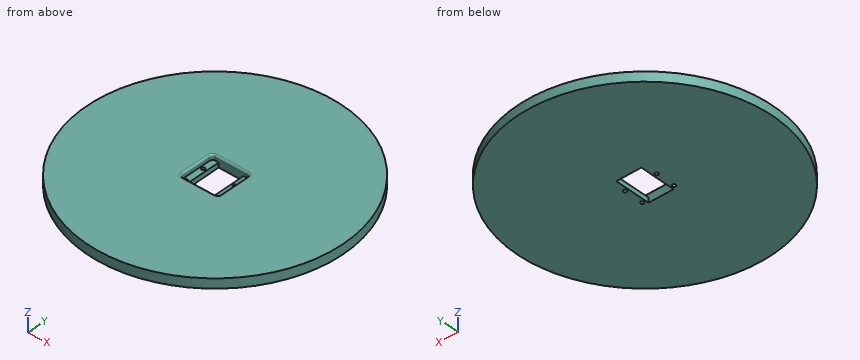
from build123d import *

# Parameters (mm, degrees)
SKETCH1_R           = 84.93125
BOSS_EXTRUDE1_DEPTH = 6.35
CUT_EXTRUDE2_DEPTH  = 3.175
SKETCH4_R           = 1.143
SKETCH4_W           = 16.6116
SKETCH4_H           = 23.7998
CUT_EXTRUDE3_DEPTH  = 3.175
FILLET1_R           = 1.27


with BuildPart() as part:
    # Sketch1 → Boss-Extrude1 (new body)
    with BuildSketch(Plane.XY):
        Circle(SKETCH1_R)
    extrude(amount=BOSS_EXTRUDE1_DEPTH)

    # Sketch2 → Cut-Extrude2 (cut)
    with BuildSketch(Plane.XY.offset(6.35)):
        with BuildLine():
            Line((10.541, 11.8999), (-10.541, 11.8999))
            ThreePointArc((-10.541, 11.8999), (-11.995801492, 11.297301492), (-12.5984, 9.8425))
            Line((-12.5984, 9.8425), (-12.5984, -9.8425))
            ThreePointArc((-12.5984, -9.8425), (-11.995801492, -11.297301492), (-10.541, -11.8999))
            Line((-10.541, -11.8999), (10.541, -11.8999))
            ThreePointArc((10.541, -11.8999), (11.995801492, -11.297301492), (12.5984, -9.8425))
            Line((12.5984, -9.8425), (12.5984, 9.8425))
            ThreePointArc((12.5984, 9.8425), (11.995801492, 11.297301492), (10.541, 11.8999))
        make_face()
    extrude(amount=-CUT_EXTRUDE2_DEPTH, mode=Mode.SUBTRACT)

    # Sketch4 → Cut-Extrude3 (cut)
    with BuildSketch(Plane.XY.offset(3.175)):
        with Locations((10.541, -9.8425)):
            Circle(SKETCH4_R)
        with Locations((-10.541, -9.8425)):
            Circle(SKETCH4_R)
        with Locations((10.541, 2.9845)):
            Circle(SKETCH4_R)
        with Locations((-10.541, 2.9845)):
            Circle(SKETCH4_R)
        Rectangle(SKETCH4_W, SKETCH4_H)
    extrude(amount=-CUT_EXTRUDE3_DEPTH, mode=Mode.SUBTRACT)

    # Fillet1
    fillet1_edges = [part.edges().sort_by_distance(p)[0] for p in [
        (-12.5984, 0, 6.35),
        (11.995801492, -11.297301492, 6.35),
        (12.5984, 0, 6.35),
        (11.995801492, 11.297301492, 6.35),
        (-11.995801492, -11.297301492, 6.35),
        (0, -11.8999, 6.35),
        (0, 11.8999, 6.35),
        (-11.995801492, 11.297301492, 6.35),
    ]]
    fillet(fillet1_edges, radius=FILLET1_R)


solid = part.part
Input: part model. Units: mm. Frame: model coordinates. Round coordinates to 2 decimals unless told otherwise and drop trailing zeros. Order: outer loops, then holes, each group sorted by start corner. A loop starts at its lowest first (then second) coordinate and runs counter-clockwise, first axis right, second up.
1. Cut plane C-C, the plane y = -53. Output: boundary loops of the cut face in (x, z).
The answers:
outline: (-66.37, 0) - (66.37, 0) - (66.37, 6.35) - (-66.37, 6.35) - close
2. Pin query (flat end, axial travel): P1, Ø1.6, axis at y = 1.5, z = 1.5, coming from the -X side; P2, Ø3, axis at x = -10.54, y = 2.98, coming from the +Z side (3 decimals); P3, Ø1.6, axis at y = -2, z = 2.5, coming from the +X side. Return the tip coordinate at first contact, or that it passes through.
The answers:
P1: stops at x = -84.93
P2: stops at z = 3.175
P3: stops at x = 84.92
3. Material intervals for line 1 (Z direction, x = -12, y = -8.5) (3 decimals); line 2 (Y direction, x = -6, z = 6); line 3 (Y direction, x = -75, z = 3.5), sorted ascending.
The answers:
line 1: z = 0 to 3.175
line 2: y = -84.72 to -12.29, 12.29 to 84.72
line 3: y = -39.85 to 39.85
4. Cut plane B-B, the plane z = 1.25. Output: boundary loops of the cut face in (x, y).
The answers:
outline: circle Ø169.86 at (0, 0); hole circle Ø2.29 at (-10.54, -9.84); hole circle Ø2.29 at (-10.54, 2.98); hole (-8.31, -11.9) - (8.31, -11.9) - (8.31, 11.9) - (-8.31, 11.9) - close; hole circle Ø2.29 at (10.54, -9.84); hole circle Ø2.29 at (10.54, 2.98)
5. Cut plane A-A, the plane x = 0. Output: boundary loops of the cut face in (y, z).
The answers:
outline: (-84.93, 0) - (-11.9, 0) - (-11.9, 5.08) arc R1.27 ccw to (-13.17, 6.35) - (-84.93, 6.35) - close; (11.9, 0) - (84.93, 0) - (84.93, 6.35) - (13.17, 6.35) arc R1.27 ccw to (11.9, 5.08) - close
6. Cut plane D-D, the plane x = 64. Output: boundary loops of the cut face in (y, z), then the cut area to 3 significant figures.
The answers:
outline: (-55.83, 0) - (55.83, 0) - (55.83, 6.35) - (-55.83, 6.35) - close
area: 709 mm2
